Design review of the part built by this model. Coordinates are the model's own, in mm. Round coordinates to 2 decimals unless told otherwise and drop trailing zeros. Order: outer loops, then holes, each group sorted by start corner. A loop starts at its lowest first (then second) coordinate and runs counter-clockwise, first axis right, second up. Notation, with made-up numbers: (85.25, 21.25) - (127.25, 21.25) arc R21 cw to (127.25, 57.25) - close; hole circle Ø6 at (67, 20). An arc over 180 degrees is marked (long way). Write item = value, one per line.
from build123d import *
from OCP.BRepFilletAPI import BRepFilletAPI_MakeChamfer

# Parameters (mm, degrees)
BOSS_EXTRUDE1_DEPTH = 4
CHAMFER2_SIZE       = 2
CHAMFER2_SIZE2      = 2.02259675


with BuildPart() as part:
    # Sketch2 → Boss-Extrude1 (new body)
    with BuildSketch(Plane(origin=(0, 0, 0), x_dir=(1, 0, 0), z_dir=(0, 1, 0))):
        Polygon((0, 9), (45, 8.5), (45, 0.5), (0, 0), align=None)
    extrude(amount=BOSS_EXTRUDE1_DEPTH)

    # Chamfer2: one chamfer whose edges measure the first distance from different faces: ONE call of the kernel's chamfer builder (chamfer() names one face for all edges)
    chamfer2_edges_1 = [part.edges().sort_by_distance(p)[0] for p in [
        (45, 2, -8.5),
    ]]
    chamfer2_side_1 = [part.faces().sort_by_distance(p)[0] for p in [
        (45, 2, -4.5),
    ]]
    chamfer2_edges_2 = [part.edges().sort_by_distance(p)[0] for p in [
        (45, 2, -0.5),
    ]]
    chamfer2_side_2 = [part.faces().sort_by_distance(p)[0] for p in [
        (22.5, 2, -0.25),
    ]]
    chamfer2 = BRepFilletAPI_MakeChamfer(part.part.solid().wrapped)
    for e in chamfer2_edges_1:
        chamfer2.Add(CHAMFER2_SIZE, CHAMFER2_SIZE2, e.wrapped, chamfer2_side_1[0].wrapped)  # the first distance lies on this face
    for e in chamfer2_edges_2:
        chamfer2.Add(CHAMFER2_SIZE, CHAMFER2_SIZE2, e.wrapped, chamfer2_side_2[0].wrapped)  # the first distance lies on this face
    add(Compound.cast(chamfer2.Shape()), mode=Mode.REPLACE)


solid = part.part
1) The part is to be moulded in two halves that separate along X. For faces 1 (the flat face through (23, 0, -5)), 2 (the flat face through (0, 2, -4)), 3 (the flat face through (44, 2, -7.5)), say which applies: released by +X, released by -X, zero draft, split by the parting line, or undercut.
Findings:
face_1 = zero draft
face_2 = released by -X
face_3 = released by +X
2) We need section B-B on x = 38.5. Write out the cut boundary in (y, z), and give its area (3 significant figures).
Findings:
outline = (0, -8.57) - (4, -8.57) - (4, -0.43) - (0, -0.43) - close
area = 32.6 mm^2
3) We need section C-C on z = -1.25. Write out the cut boundary in (x, y).
Findings:
outline = (0, 0) - (43.76, 0) - (43.76, 4) - (0, 4) - close
4) We need section A-A on y = 2.5. Write out the cut boundary in (x, z).
Findings:
outline = (0, -9) - (42.98, -8.52) - (45, -6.5) - (45, -2.52) - (43, -0.48) - (0, 0) - close
5) Clearance check with flat-ended pins moving along their axes: pin 1 Ø1 at (x, y) = (15.5, 1) entering from -Z; pin 2 Ø1.5 at (x, y) = (34.5, 2.5) entering from -Z (3 decimals). State where each tip first meets the part, or that it passes through.
Findings:
pin_1 = -8.83
pin_2 = -8.625
6) To check wall thickness, follow L1, parallel to X at y = 0.75, z = -8; L2, parallel to X at y = 1.9, z = -1.25; L3, parallel to Z at x = 18.5, y = 3.55. State the ranges of each line that lie inside material, in increasing order. Write a range as from..to.
Findings:
L1 = 0..43.5
L2 = 0..43.76
L3 = -8.79..-0.21
